CAD build for the part. Positions are in the model's coordinates, mm. A direction names the side the tool comes from. Coordinates: 2 decimals unless noted, no trailing zeros. Order: outer loops, then holes, each group sorted by start corner. A loop starts at its lowest first (then second) coordinate and runs counter-clockwise, first axis right, second up. Notation, with made-up numbers: M 52,-10.5 L 89,-10.5 A14 cw 89,6.5 Z; hole C 6,85 d5. An arc over 180 degrees is marked long. One line per item, written item: value.
from build123d import *

# Parameters (mm, degrees)
BOSS_EXTRUDE1_DEPTH = 6.35
SKETCH3_W           = 28.575
SKETCH3_H           = 22.86
BOSS_EXTRUDE2_DEPTH = 52.8
SKETCH6_W           = 28.575
SKETCH6_H           = 100
BOSS_EXTRUDE3_DEPTH = 5.08
FILLET1_R           = 5.08
SKETCH4_W           = 6.35
SKETCH4_H           = 24.225
SKETCH4_W_2         = 11.049
CUT_EXTRUDE1_DEPTH  = 153.525464126
FILLET3_R           = 11.43
SKETCH5_R           = 6.604
CUT_EXTRUDE2_DEPTH  = 157.642486403


with BuildPart() as part:
    # Sketch1 → Boss-Extrude1 (new body)
    with BuildSketch(Plane.XY):
        Polygon((-18.271216857, 45), (18.271216857, 45), (61.572487047, 120), (78.070270989, 110.475), (14.2875, 0), (14.2875, -100), (-14.2875, -100), (-14.2875, 0), (-78.070270989, 110.475), (-61.572487047, 120), align=None)
    extrude(amount=BOSS_EXTRUDE1_DEPTH)

    # Sketch3 → Boss-Extrude2 (add)
    with BuildSketch(Plane.XY.offset(6.35)):
        with Locations((0, 11.43)):
            Rectangle(SKETCH3_W, SKETCH3_H)
    extrude(amount=BOSS_EXTRUDE2_DEPTH)

    # Sketch6 → Boss-Extrude3 (add)
    with BuildSketch(Plane.XY.offset(6.35)):
        with Locations((0, -50)):
            Rectangle(SKETCH6_W, SKETCH6_H)
    extrude(amount=BOSS_EXTRUDE3_DEPTH)

    # Fillet1
    fillet1_edges = [part.edges().sort_by_distance(p)[0] for p in [
        (-18.271216857, 45, 3.175),
        (18.271216857, 45, 3.175),
        (61.572487047, 120, 3.175),
        (78.070270989, 110.475, 3.175),
        (14.2875, 0, 3.175),
        (14.2875, -100, 5.715),
        (-14.2875, -100, 5.715),
        (-14.2875, 0, 3.175),
        (-78.070270989, 110.475, 3.175),
        (-61.572487047, 120, 3.175),
    ]]
    fillet(fillet1_edges, radius=FILLET1_R)

    # Sketch4 → Cut-Extrude1 (cut, through all)
    with BuildSketch(Plane.XZ):
        with Locations((-11.1125, 47.0375)):
            Rectangle(SKETCH4_W, SKETCH4_H)
        with Locations((3.175, 47.0375)):
            Rectangle(SKETCH4_W_2, SKETCH4_H)
    extrude(amount=-CUT_EXTRUDE1_DEPTH, mode=Mode.SUBTRACT)

    # Fillet3
    fillet3_edges = [part.edges().sort_by_distance(p)[0] for p in [
        (11.4935, 22.86, 59.15),
        (-5.1435, 22.86, 59.15),
        (11.4935, 0, 59.15),
        (-5.1435, 0, 59.15),
    ]]
    fillet(fillet3_edges, radius=FILLET3_R - 0.0001)  # a hair under: the kernel refuses the full size

    # Sketch5 → Cut-Extrude2 (cut, through all)
    with BuildSketch(Plane.ZY.offset(7.9375)):
        with Locations(Location((47.72, 11.43, 0), (0, 0, 270))):
            Circle(SKETCH5_R)
    extrude(amount=-CUT_EXTRUDE2_DEPTH, mode=Mode.SUBTRACT)


solid = part.part
Q1. Mould opens along X. For faces 5 (the face through (0, -49, 11.43)), 6 (the face through (0, 45, 3)), 7 (the face through (76.05, 109.88, 3.22)) say: released by +X, released by -X, zero draft, split by the parting line, or undercut.
Recorded:
face 5: zero draft
face 6: undercut
face 7: released by +X
Q2. Slice it at C-C (y = 27.5). List the corners of the cut face in (x, z).
Recorded:
outline: M -30.16,0 L 30.16,0 L 30.16,6.35 L -30.16,6.35 Z
Q3. Slice it at D-D (z = 19). List the corners of the cut face in (x, y), plus the area to 3 significant figures.
Recorded:
outline: M -14.29,0 L 14.29,0 L 14.29,22.86 L -14.29,22.86 Z
area: 653 mm^2
Q4. Slice it at A-A (x = 5). List the corners of the cut face in (y, z) (3 decimals), plus the area to 3 significant figures.
Recorded:
outline: M -100,0 L 45,0 L 45,6.35 L 22.86,6.35 L 22.86,34.925 L 0,34.925 L 0,11.43 L -100,11.43 Z
area: 2,080 mm^2
Q5. Drill centre lines: line 1 along Z through (x, y) = (-3, 11); line 2 along Z through (x, y) = (-6.55, 11.43); line 3 along Y through (x, z) = (-5.5, 24). Where is each one in solid material? Low to high.
Recorded:
line 1: z = 0 to 41.13, 54.31 to 59.14
line 2: z = 0 to 41.12, 54.32 to 59.15
line 3: y = 0 to 22.86
Q6. Pin check, flat tips, straight feed: pin 1 Ø7 at (x, y) = (-11.5, 10.5) entering from +Z (3 decimals); pin 2 Ø10.5 at (y, z) = (-65, 21) entering from -X; pin 3 Ø3 at (x, z) = (3, 2.5) entering from +Y; pin 4 Ø5 at (x, z) = (12.5, 20.5) entering from +Y. Stop position of each tip, or through.
Recorded:
pin 1: stops at z = 34.925
pin 2: passes through
pin 3: stops at y = 45
pin 4: stops at y = 22.86
Q7. Which spindle directions (+Z, -Z, +X, -X, +Y, -Y) get a long thin tool onto all of the face, cutting with end or side? Do faces 1 (the face through (3, 11, 34.925)), 2 (the face through (0, 0, 25)), 3 (the face through (-7.938, 9, 41)), 4 (the face through (17.91, 45.7, 3.22)). Say none if no direction does.
Recorded:
face 1: +Z, +Y, -Y
face 2: +Z, +X, -X, -Y
face 3: +Z, -X, +Y, -Y
face 4: +Z, -Z, +Y
Q8. Slice it at B-B (z = 9). List the corners of the cut face in (x, y), plus the area to 3 significant figures.
Recorded:
outline: M -14.29,-94.92 A5.08 ccw -9.21,-100 L 9.21,-100 A5.08 ccw 14.29,-94.92 L 14.29,22.86 L -14.29,22.86 Z
area: 3,500 mm^2
